Geometry: final body of the model. Coordinates: model frame, mm. Face numbers are marked on the shaded views. A direction names the side the tool comes from. Round coordinates to 2 decimals unless told otherwise and drop trailing zeros. Loops run counter-clockwise (first coordinate to the right, second up) from the corner with the lowest first, then second, coordinate; pieces in that order, holes last. Notation, with made-up numbers: M -12,53 L 26,53 A22 cw 26,67 Z; hole C 35,29.5 d3. An arc over 180 degrees is marked long. Write each question's results on one line, items separated by ' | '.
Autodesk Inventor part; units mm, degrees
ref_plane "YZ Plane" through (0, 0, 0) normal (1, 0, 0) x (0, 1, 0)
ref_plane "XZ Plane" through (0, 0, 0) normal (0, 1, 0) x (-1, 0, 0)
ref_plane "XY Plane" through (0, 0, 0) normal (0, 0, 1) x (1, 0, 0)
sketch "Sketch1" plane through (0, 0, 0) normal (0, 0, 1) x (1, 0, 0)
  line L0 (-83.046, 15.2299) -> (66.954, 15.2299)
  line L1 (66.954, 15.2299) -> (66.954, -4.7701)
  line L2 (66.954, -4.7701) -> (-83.046, -4.7701)
  line L3 (-83.046, -4.7701) -> (-83.046, 15.2299)
  point P0 (0, 0)
  dimension "d0" = 150
  dimension "d1" = 20
extrude "Extrusion1" add sketch "Sketch1" along normal blind 10
sketch "Sketch2" plane through (-83.046, -4.7701, 0) normal (-1, 0, 0) x (0, 0, 1)
  point P0 (0, 4.7701)
sketch "Sketch3" plane through (-83.046, -4.7701, 0) normal (-1, 0, 0) x (0, 0, 1)
  line L0 (0, 20) -> (-4, 20)
  line L1 (-4, 20) -> (-4, 0)
  line L2 (-4, 0) -> (0, 0)
  line L3 (0, 0) -> (0, 20)
  line L4 (10, 0) -> (14, 0)
  line L5 (14, 0) -> (14, 20)
  line L6 (14, 20) -> (10, 20)
  line L7 (10, 20) -> (10, 0)
  line L8 (0, 0) -> (10, 0)
  line L9 (10, 20) -> (10, 0)
  point P0 (0, 4.7701)
  dimension "d4" = 4
  dimension "d5" = 4
extrude "Extrusion2" add sketch "Sketch3" against normal blind 5
sketch "Sketch4" plane through (-83.046, -4.7701, 14) normal (-1, 0, 0) x (0, 0, 1)
  line L0 (-18, 20) -> (-14, 20)
  line L1 (-14, 20) -> (-14, 0)
  line L2 (-14, 0) -> (-18, 0)
  line L3 (-18, 0) -> (-18, 20)
  line L4 (0, 20) -> (-4, 20)
  line L5 (-4, 20) -> (-4, 0)
  line L6 (-4, 0) -> (0, 0)
  line L7 (0, 0) -> (0, 20)
  point P0 (-14, 4.7701)
extrude "Extrusion3" add sketch "Sketch4" along normal blind 30
sketch "Sketch5" plane through (-78.046, -4.7701, 14) normal (0, 0, 1) x (1, 0, 0)
  line L0 (-35, 0) -> (-35, 20)
  line L1 (-5, 20) -> (-35, 20)
  line L2 (-5, 0) -> (-5, 20)
  point P0 (78.046, 4.7701)
  point P1 (-30, 15)
  point P2 (-10, 15)
  dimension "d10" = 5
  dimension "d11" = 5
  dimension "d12" = 5
  dimension "d13" = 5
hole "Hole1" at (-108.046, 10.2299, 14) at (-88.046, 10.2299, 14) direction (0, 0, -1) diameter 3 depth 30 tip angle 118 countersink diameter 6 countersink angle 90
chamfer "Chamfer1" distance 4 angle 45 2 edges at (-78.046, 5.2299, 10) (-78.046, 5.2299, 0)
sketch "Sketch6" plane through (66.954, -4.7701, 0) normal (0, -1, 0) x (1, 0, 0)
  line L0 (0, -4) -> (-5, -4)
  line L1 (-5, -4) -> (-5, 14)
  line L2 (-5, 14) -> (0, 14)
  line L3 (0, 14) -> (0, -4)
  line L4 (0, 0) -> (-141, 0)
  line L5 (-141, 10) -> (0, 10)
  line L6 (0, 0) -> (0, 10)
  point P0 (-66.954, 0)
  dimension "d24" = 4
  dimension "d25" = 4
  dimension "d26" = 5
extrude "Extrusion4" add sketch "Sketch6" against normal blind 20
sketch "Sketch7" plane through (-113.046, -4.7701, 10) normal (0, -1, 0) x (1, 0, 0)
  line L0 (180, -14) -> (210, -14)
  line L1 (210, -14) -> (210, -10)
  line L2 (210, -10) -> (180, -10)
  line L3 (180, -10) -> (180, -14)
  line L4 (180, 4) -> (210, 4)
  line L5 (210, 4) -> (210, 0)
  line L6 (210, 0) -> (180, 0)
  line L7 (180, 0) -> (180, 4)
  point P0 (113.046, -10)
  dimension "d29" = 30
  dimension "d30" = 30
  dimension "d31" = 4
  dimension "d32" = 4
extrude "Extrusion5" add sketch "Sketch7" against normal blind 20
chamfer "Chamfer2" distance 4 angle 45 2 edges at (61.954, 5.2299, 10) (61.954, 5.2299, 0)
sketch "Sketch8" plane through (96.954, -4.7701, 14) normal (0, 0, 1) x (1, 0, 0)
  line L0 (-30, 20) -> (-30, 0)
  line L1 (0, 0) -> (0, 20)
  line L2 (-35, 20) -> (0, 20)
  line L3 (-35, 0) -> (0, 0)
  circle A0 centre (-25, 5) radius 2
  circle A1 centre (-25, 15) radius 2
  circle A2 centre (-5, 5) radius 2
  circle A3 centre (-5, 15) radius 2
  line L4 (-25, 3) -> (-5, 3)
  line L5 (-5, 7) -> (-25, 7)
  line L6 (-25, 13) -> (-5, 13)
  line L7 (-5, 17) -> (-25, 17)
  point P0 (-96.954, 4.7701)
  dimension "d38" = 5
  dimension "d39" = 5
  dimension "d40" = 5
  dimension "d41" = 5
  dimension "d42" = 5
  dimension "d43" = 5
  dimension "d44" = 5
  dimension "d45" = 5
  dimension "d46" = 4
  dimension "d47" = 4
  dimension "d48" = 4
  dimension "d49" = 4
extrude "Extrusion6" cut sketch "Sketch8" against normal blind 20 contours A0 | A0 L5 A2 L4 | A2 | A1 | A1 L7 A3 L6 | A3
properties part number "Upper Support beam"
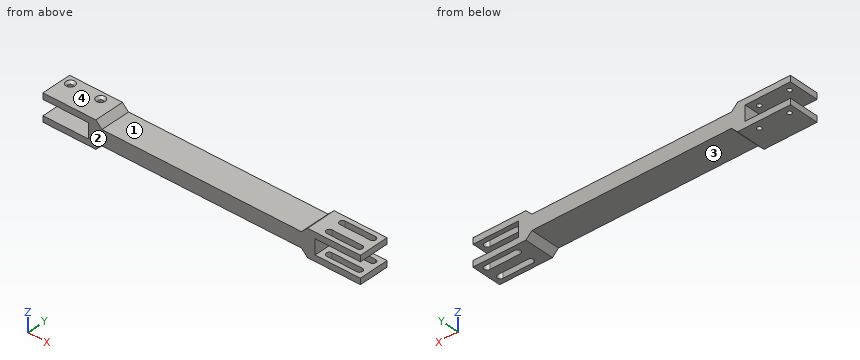
1. Draft query along X for the marked faces 3 and 4. Return one class per face: pulls with the +X half, pulls with the -X half, needs draft (parallel to the pull), parting line crosses it, or undercut.
Answer key:
face 3: undercut | face 4: needs draft
2. Access query for the marked faces 1 and 2. Directions: +Z, -Z, +X, -X, +Y, -Y. A direction counts if a zero-diameter tool reaches every point of the face in a straight line with its end or side. Return the directions, or none.
Answer key:
face 1: +Z, +Y, -Y | face 2: +Z, -Z, +X, -X, -Y
3. Section B-B (z = -2). Output: boundary loops of the cut face in (x, y), then the cut area to 3 significant figures.
Answer key:
outline: M -113.05,-4.77 L -76.05,-4.77 L -76.05,15.23 L -113.05,15.23 Z; M 59.95,-4.77 L 96.95,-4.77 L 96.95,15.23 L 59.95,15.23 Z; hole C -108.05,10.23 d3; hole C -88.05,10.23 d3; hole M 71.95,-1.77 L 91.95,-1.77 A2 ccw 91.95,2.23 L 71.95,2.23 A2 ccw Z; hole M 71.95,8.23 L 91.95,8.23 A2 ccw 91.95,12.23 L 71.95,12.23 A2 ccw Z | area: 1,280 mm²
4. Pin query (flat end, axial travel): P1, Ø5, axis at y = 10, z = 3.5, coming from the +X side; P2, Ø3, axis at y = 2, z = 2, coming from the -X side; P3, Ø8, axis at x = -20.5, y = 7.5, coming from the +Z side. Return the tip coordinate at first contact, or that it passes through.
Answer key:
P1: stops at x = 66.95 | P2: stops at x = -83.05 | P3: stops at z = 10
5. Section A-A (x = -98). Output: boundary loops of the cut face in (y, z).
Answer key:
outline: M -4.77,-4 L 15.23,-4 L 15.23,0 L -4.77,0 Z; M -4.77,10 L 15.23,10 L 15.23,14 L -4.77,14 Z
6. Ray query, probe 1 along Z at (x, y) = (-97, 5.75); probe 2 along X at (y, z) = (12, 10.75) (1 decimal); probe 3 along X at (y, z) = (2, -2.75) (1 decimal). Return the intervals inside material, ascending.
Answer key:
probe 1: z = -4 to 0, 10 to 14 | probe 2: x = -113 to -74.8, 58.7 to 71, 92.9 to 97 | probe 3: x = -113 to -76.8, 60.7 to 71, 92.9 to 97
7. Section C-C (x = -50). Output: boundary loops of the cut face in (y, z).
Answer key:
outline: M -4.77,0 L 15.23,0 L 15.23,10 L -4.77,10 Z
8. Section D-D (z = 8). Output: boundary loops of the cut face in (x, y).
Answer key:
outline: M -83.05,-4.77 L 66.95,-4.77 L 66.95,15.23 L -83.05,15.23 Z
